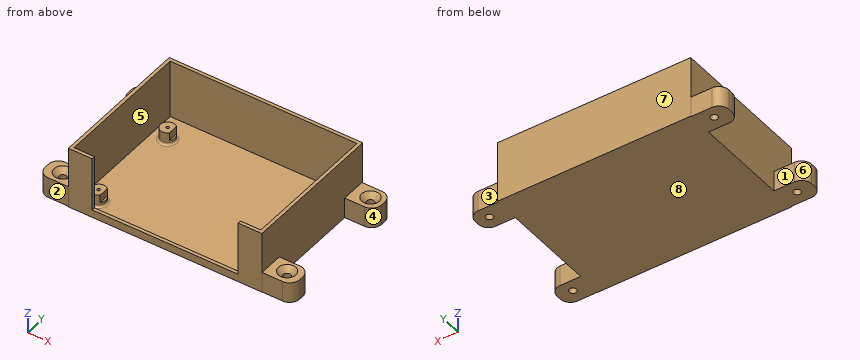
```python
from build123d import *

# Parameters (mm, degrees)
BOX001_W          = 71
BOX001_H          = 67
BOX001_DEPTH      = 30
CYLINDER001_R     = 1.5
CYLINDER001_DEPTH = 10
CYLINDER002_R     = 1.5
CYLINDER002_DEPTH = 10
CYLINDER003_R     = 1.5
CYLINDER003_DEPTH = 10
CYLINDER_R        = 1.5
CYLINDER_DEPTH    = 10
BOX_W             = 86
BOX_H             = 58
BOX_DEPTH         = 1.5
BOX002_W          = 94
BOX002_H          = 70
BOX002_DEPTH      = 30
THICKNESS_T       = -1.6
CYLINDER005_R     = 0.75
CYLINDER005_DEPTH = 10
CYLINDER004_R     = 3.5
CYLINDER004_DEPTH = 6
CYLINDER007_R     = 0.75
CYLINDER007_DEPTH = 10
CYLINDER006_R     = 3.5
CYLINDER006_DEPTH = 6
CYLINDER009_R     = 0.75
CYLINDER009_DEPTH = 10
CYLINDER008_R     = 3.5
CYLINDER008_DEPTH = 6
CYLINDER010_R     = 0.75
CYLINDER010_DEPTH = 10
CYLINDER011_R     = 3.5
CYLINDER011_DEPTH = 6
FILLET_R          = 1
FILLET001_R       = 1
CYLINDER014_R     = 1.75
CYLINDER014_DEPTH = 20
CYLINDER013_R     = 1.75
CYLINDER013_DEPTH = 20
CYLINDER015_R     = 1.75
CYLINDER015_DEPTH = 20
CYLINDER012_R     = 1.75
CYLINDER012_DEPTH = 20
BOX004_W          = 15
BOX004_H          = 12
BOX004_DEPTH      = 10
BOX005_W          = 15
BOX005_H          = 12
BOX005_DEPTH      = 10
BOX006_W          = 15
BOX006_H          = 12
BOX006_DEPTH      = 10
BOX003_W          = 15
BOX003_H          = 12
BOX003_DEPTH      = 10
FILLET002_R       = 4.9
FILLET003_R       = 4.9
CHAMFER_SIZE      = 2.5


with BuildPart() as obj1:
    # Box001 → Box001 (new body)
    with BuildSketch(Plane(origin=(7.49857, 58.9, 26), x_dir=(1, 0, 0), z_dir=(0, 0, -1))):
        with Locations((35.5, 33.5)):
            Rectangle(BOX001_W, BOX001_H)
    extrude(amount=BOX001_DEPTH)


with BuildPart() as zylinder001:
    # Cylinder001 → Cylinder001 (new body)
    with BuildSketch(Plane(origin=(5, 53, 0), x_dir=(1, 0, 0), z_dir=(0, 0, 1))):
        Circle(CYLINDER001_R)
    extrude(amount=CYLINDER001_DEPTH)


with BuildPart() as zylinder002:
    # Cylinder002 → Cylinder002 (new body)
    with BuildSketch(Plane(origin=(81.5, 5, 0), x_dir=(1, 0, 0), z_dir=(0, 0, 1))):
        Circle(CYLINDER002_R)
    extrude(amount=CYLINDER002_DEPTH)


with BuildPart() as zylinder003:
    # Cylinder003 → Cylinder003 (new body)
    with BuildSketch(Plane(origin=(81.5, 53, 0), x_dir=(1, 0, 0), z_dir=(0, 0, 1))):
        Circle(CYLINDER003_R)
    extrude(amount=CYLINDER003_DEPTH)


with BuildPart() as fusion:
    # Cylinder → Cylinder (new body)
    with BuildSketch(Plane(origin=(5, 5, 0), x_dir=(1, 0, 0), z_dir=(0, 0, 1))):
        Circle(CYLINDER_R)
    extrude(amount=CYLINDER_DEPTH)

    # Fusion: union Zylinder001, Zylinder002, Zylinder003
    add(zylinder001.part)
    add(zylinder002.part)
    add(zylinder003.part)


with BuildPart() as fusion001:
    # Box → Box (new body)
    with BuildSketch(Plane.XY):
        with Locations((43, 29)):
            Rectangle(BOX_W, BOX_H)
    extrude(amount=BOX_DEPTH)

    # Cut: cut Fusion
    add(fusion.part, mode=Mode.SUBTRACT)

    # Fusion001: union obj1
    add(obj1.part)


with BuildPart() as fusion001_1:
    # Fusion001 placement: moved
    add(fusion001.part.moved(Location((0, -5, 2.8))))


with BuildPart() as thickness:
    # Box002 → Box002 (new body)
    with BuildSketch(Plane(origin=(-4.00143, -8.1, -5), x_dir=(1, 0, 0), z_dir=(0, 0, 1))):
        with Locations((47, 35)):
            Rectangle(BOX002_W, BOX002_H)
    extrude(amount=BOX002_DEPTH)

    # Thickness
    thickness_openings = [thickness.faces().sort_by_distance(p)[0] for p in [
        (42.99857, 26.9, 25),
    ]]
    offset(amount=THICKNESS_T, openings=thickness_openings)


with BuildPart() as zylinder005:
    # Cylinder005 → Cylinder005 (new body)
    with BuildSketch(Plane(origin=(5, 0, -6), x_dir=(1, 0, 0), z_dir=(0, 0, 1))):
        Circle(CYLINDER005_R)
    extrude(amount=CYLINDER005_DEPTH)


with BuildPart() as cut001:
    # Cylinder004 → Cylinder004 (new body)
    with BuildSketch(Plane(origin=(5, 0, -3.4), x_dir=(1, 0, 0), z_dir=(0, 0, 1))):
        Circle(CYLINDER004_R)
    extrude(amount=CYLINDER004_DEPTH)

    # Cut001: cut Zylinder005
    add(zylinder005.part, mode=Mode.SUBTRACT)


with BuildPart() as zylinder007:
    # Cylinder007 → Cylinder007 (new body)
    with BuildSketch(Plane(origin=(5, 0, -6), x_dir=(1, 0, 0), z_dir=(0, 0, 1))):
        Circle(CYLINDER007_R)
    extrude(amount=CYLINDER007_DEPTH)


with BuildPart() as cut002:
    # Cylinder006 → Cylinder006 (new body)
    with BuildSketch(Plane(origin=(5, 0, -3.4), x_dir=(1, 0, 0), z_dir=(0, 0, 1))):
        Circle(CYLINDER006_R)
    extrude(amount=CYLINDER006_DEPTH)

    # Cut002: cut Zylinder007
    add(zylinder007.part, mode=Mode.SUBTRACT)


with BuildPart() as cut002_1:
    # Cut002 placement: moved
    add(cut002.part.moved(Location((0, 48, 0))))


with BuildPart() as zylinder009:
    # Cylinder009 → Cylinder009 (new body)
    with BuildSketch(Plane(origin=(5, 0, -6), x_dir=(1, 0, 0), z_dir=(0, 0, 1))):
        Circle(CYLINDER009_R)
    extrude(amount=CYLINDER009_DEPTH)


with BuildPart() as cut003:
    # Cylinder008 → Cylinder008 (new body)
    with BuildSketch(Plane(origin=(5, 0, -3.4), x_dir=(1, 0, 0), z_dir=(0, 0, 1))):
        Circle(CYLINDER008_R)
    extrude(amount=CYLINDER008_DEPTH)

    # Cut003: cut Zylinder009
    add(zylinder009.part, mode=Mode.SUBTRACT)


with BuildPart() as cut003_1:
    # Cut003 placement: moved
    add(cut003.part.moved(Location((76.5, 48, 0))))


with BuildPart() as zylinder010:
    # Cylinder010 → Cylinder010 (new body)
    with BuildSketch(Plane(origin=(5, 0, -6), x_dir=(1, 0, 0), z_dir=(0, 0, 1))):
        Circle(CYLINDER010_R)
    extrude(amount=CYLINDER010_DEPTH)


with BuildPart() as fillet001:
    # Cylinder011 → Cylinder011 (new body)
    with BuildSketch(Plane(origin=(5, 0, -3.4), x_dir=(1, 0, 0), z_dir=(0, 0, 1))):
        Circle(CYLINDER011_R)
    extrude(amount=CYLINDER011_DEPTH)

    # Cut004: cut Zylinder010
    add(zylinder010.part, mode=Mode.SUBTRACT)


with BuildPart() as fillet001_1:
    # Cut004 placement: moved
    add(fillet001.part.moved(Location((76.5, 0, 0))))

    # Fusion002: union Cut001, Cut002, Cut003
    add(cut001.part)
    add(cut002_1.part)
    add(cut003_1.part)

    # Fusion003: union Thickness
    add(thickness.part)

    # Fillet
    fillet_edges = [fillet001_1.edges().sort_by_distance(p)[0] for p in [
        (1.5, 48, -3.4),
        (78, 48, -3.4),
    ]]
    fillet(fillet_edges, radius=FILLET_R)

    # Fillet001
    fillet001_edges = [fillet001_1.edges().sort_by_distance(p)[0] for p in [
        (1.5, 0, -3.4),
        (78, 0, -3.4),
    ]]
    fillet(fillet001_edges, radius=FILLET001_R)


with BuildPart() as zylinder014:
    # Cylinder014 → Cylinder014 (new body)
    with BuildSketch(Plane(origin=(98.2, 55.6, -5), x_dir=(1, 0, 0), z_dir=(0, 0, 1))):
        Circle(CYLINDER014_R)
    extrude(amount=CYLINDER014_DEPTH)


with BuildPart() as zylinder013:
    # Cylinder013 → Cylinder013 (new body)
    with BuildSketch(Plane(origin=(97.7, -1.6, -5), x_dir=(1, 0, 0), z_dir=(0, 0, 1))):
        Circle(CYLINDER013_R)
    extrude(amount=CYLINDER013_DEPTH)


with BuildPart() as zylinder015:
    # Cylinder015 → Cylinder015 (new body)
    with BuildSketch(Plane(origin=(-11.2, 55.9, -5), x_dir=(1, 0, 0), z_dir=(0, 0, 1))):
        Circle(CYLINDER015_R)
    extrude(amount=CYLINDER015_DEPTH)


with BuildPart() as fusion004:
    # Cylinder012 → Cylinder012 (new body)
    with BuildSketch(Plane(origin=(-11.2, -1.7, -5), x_dir=(1, 0, 0), z_dir=(0, 0, 1))):
        Circle(CYLINDER012_R)
    extrude(amount=CYLINDER012_DEPTH)

    # Fusion004: union Zylinder014, Zylinder013, Zylinder015
    add(zylinder014.part)
    add(zylinder013.part)
    add(zylinder015.part)


with BuildPart() as obj2:
    # Box004 → Box004 (new body)
    with BuildSketch(Plane(origin=(-18.9, 49.6, -5), x_dir=(1, 0, 0), z_dir=(0, 0, 1))):
        with Locations((7.5, 6)):
            Rectangle(BOX004_W, BOX004_H)
    extrude(amount=BOX004_DEPTH)


with BuildPart() as obj3:
    # Box005 → Box005 (new body)
    with BuildSketch(Plane(origin=(89.9, -8, -5), x_dir=(1, 0, 0), z_dir=(0, 0, 1))):
        with Locations((7.5, 6)):
            Rectangle(BOX005_W, BOX005_H)
    extrude(amount=BOX005_DEPTH)


with BuildPart() as obj4:
    # Box006 → Box006 (new body)
    with BuildSketch(Plane(origin=(89.5, 49.4, -5), x_dir=(1, 0, 0), z_dir=(0, 0, 1))):
        with Locations((7.5, 6)):
            Rectangle(BOX006_W, BOX006_H)
    extrude(amount=BOX006_DEPTH)


with BuildPart() as cut006:
    # Box003 → Box003 (new body)
    with BuildSketch(Plane(origin=(-18.9, -7.8, -5), x_dir=(1, 0, 0), z_dir=(0, 0, 1))):
        with Locations((7.5, 6)):
            Rectangle(BOX003_W, BOX003_H)
    extrude(amount=BOX003_DEPTH)

    # Fusion005: union obj2, obj3, obj4
    add(obj2.part)
    add(obj3.part)
    add(obj4.part)

    # Cut005: cut Fusion004
    add(fusion004.part, mode=Mode.SUBTRACT)

    # Fusion006: union Fillet001
    add(fillet001_1.part)

    # Fillet002
    fillet002_edges = [cut006.edges().sort_by_distance(p)[0] for p in [
        (-18.9, -7.8, 0),
        (-18.9, 4.2, 0),
        (-18.9, 61.6, 0),
        (-18.9, 49.6, 0),
    ]]
    fillet(fillet002_edges, radius=FILLET002_R)

    # Fillet003
    fillet003_edges = [cut006.edges().sort_by_distance(p)[0] for p in [
        (104.9, -8, 0),
        (104.9, 4, 0),
        (104.5, 61.4, 0),
        (104.5, 49.4, 0),
    ]]
    fillet(fillet003_edges, radius=FILLET003_R)

    # Chamfer
    chamfer_edges = [cut006.edges().sort_by_distance(p)[0] for p in [
        (-12.95, 55.9, 5),
        (-12.95, -1.7, 5),
        (96.45, 55.6, 5),
        (95.95, -1.6, 5),
    ]]
    chamfer(chamfer_edges, length=CHAMFER_SIZE)

    # Cut006: cut Fusion001
    add(fusion001_1.part, mode=Mode.SUBTRACT)


solid = cut006.part
```
Part model, mm, in its own coordinate system. Face numbers are marked on the shaded views. A direction names the side the tool comes from. Round coordinates to 2 decimals unless told otherwise and drop trailing zeros. Write each loop counter-clockwise with the first axis right and the second up, starting at its lowest first coordinate (ties: lowest second). Pieces come first, ordered by that corner, then holes. Notation, with made-up numbers: (-9, -34) -> (46, -34) arc R12 cw to (46, -29) -> close; hole circle Ø2 at (83.25, 13.25). An arc over 180 degrees is marked (long way). Return JSON: item names as keys, results as strings. Group by question number.
Q1. Saw through at B-B on z = 23.25. Write the cut outline in (x, y), plus the area to 3 significant figures.
Q2. Pin check, flat tips, straight feed: pin 1 (6.5 mm diameter, centred on x = 3.5, y = 47, fed in from +Z); pin 2 (8.5 mm diameter, centred on x = 60, z = 11.5, fed in from -Y); pin 3 (2.5 mm diameter, centred on y = 55.5, z = 0, fed in from +X). Stop position of each tip, or through.
Q3. Saw through at C-C on x = 70.5. Write the cut outline in (y, z), plus the area to 3 significant figures.
Q4. Probe L1, parallel to Y at x = 81.5, z = 0.15; L2, parallel to X at y = -3.5, z = 21; L3, parallel to Y at x = 3, z = 19.75. List the from-to ranges inside material, lowest first. Write a range as [from, to].
Q5. Mould opens along Y. For the marked faces 6, 7 and 8 say: pulls with the +Y half, pulls with the -Y half, needs draft (parallel to the pull), parting line crosses it, or undercut.
Q6. Saw through at A-A on y = 35. Write the cut outline in (x, z), plus the area to 3 significant figures.
Q7. Saw through at D-D on x = 97.7. State how many separate pieces and enclosed holes the cut face has, plus the area to 3 significant figures.
Q8. Which spindle directions (+Z, -Z, +X, -X, +Y, -Y) get a long thin tool onto all of the face, cutting with end or side? Do the marked faces 1, 2, 3, 4 and 5. Say none if no direction does.
Answer:
{
 "1": {"outline": "(-4, -8.1) -> (7.5, -8.1) -> (7.5, -6.5) -> (-2.4, -6.5) -> (-2.4, 60.3) -> (88.4, 60.3) -> (88.4, -6.5) -> (78.5, -6.5) -> (78.5, -8.1) -> (90, -8.1) -> (90, 61.9) -> (-4, 61.9) -> close", "area": "401 mm2"},
 "2": {"pin 1": "z = 2.6", "pin 2": "y = 60.3", "pin 3": "x = 104.5"},
 "3": {"outline": "(-8.1, -5) -> (61.9, -5) -> (61.9, 25) -> (60.3, 25) -> (60.3, -3.4) -> (-6.5, -3.4) -> (-6.5, -1.2) -> (-8.1, -1.2) -> close", "area": "161 mm2"},
 "4": {"L1": "[-8.1, -6.5], [-3.5, -0.75], [0.75, 3.5], [44.5, 47.25], [48.75, 51.5], [60.3, 61.9]", "L2": "[-4, -2.4], [88.4, 90]", "L3": "[-8.1, -6.5], [60.3, 61.9]"},
 "5": {"face 6": "undercut", "face 7": "pulls with the +Y half", "face 8": "needs draft"},
 "6": {"outline": "(-4, -5) -> (90, -5) -> (90, 25) -> (88.4, 25) -> (88.4, -3.4) -> (-2.4, -3.4) -> (-2.4, 25) -> (-4, 25) -> close", "area": "241 mm2"},
 "7": {"separate pieces": "4", "enclosed holes": "0", "area": "159 mm2"},
 "8": {"face 1": "+Z, -Z, -X", "face 2": "+Z, -Z, -X, -Y", "face 3": "+Z, -Z, +X, +Y", "face 4": "+Z, -Z, +X", "face 5": "+Z"}
}
